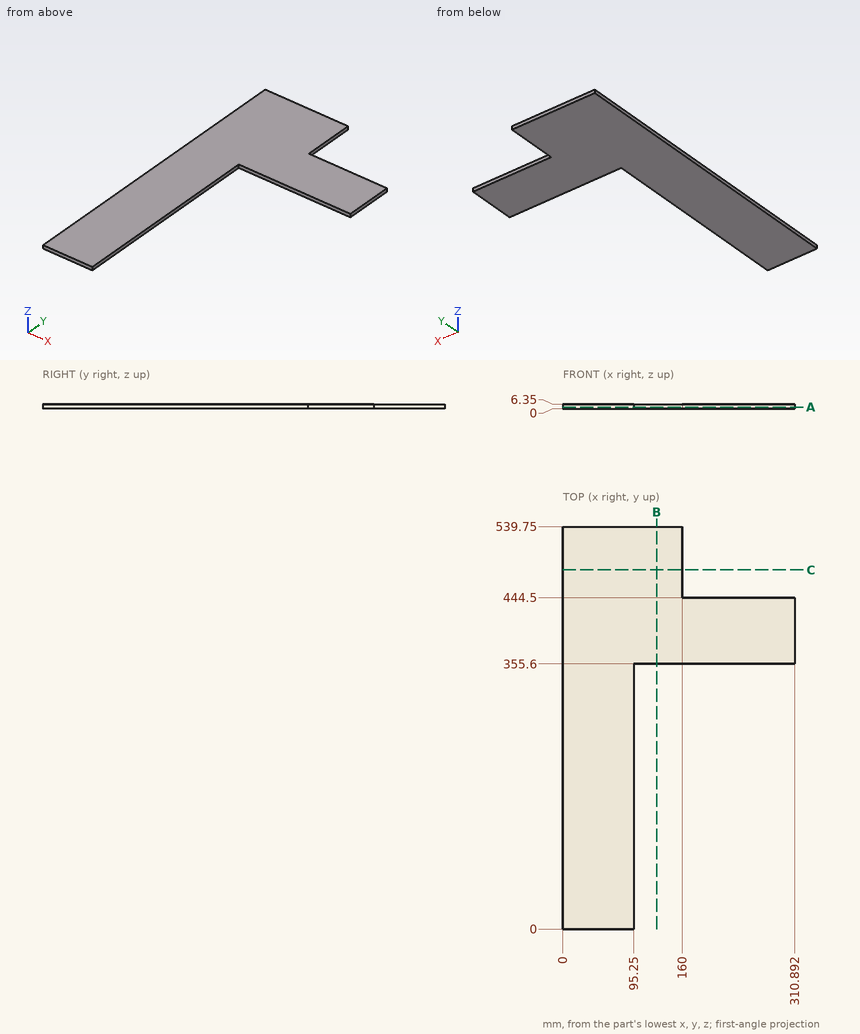
The figure shows three views and two pictorial views of one solid part (mm, origin at its lowest corner). Answer the questions. Coordinates: 2 decimals unless noted, no trailing zeros. Write each loop counter-clockwise with the first axis right and the second up, starting at its lowest first coordinate (ties: lowest second). Pieces come first, ordered by that corner, then holes. Notation, with made-up numbers: (-24, 86.5) -> (-19, 86.5) arc R10 ccw to (-19, 95.5) -> close; hole circle Ø2 at (-25, 28.5). An arc over 180 degrees is marked (long way). Answer as a JSON object with one key per item and string values.
Q1. The part is cut by section A-A on z = 2.25. Give the vertices of the cut face in (x, y).
The answers:
{"outline": "(0, 0) -> (95.25, 0) -> (95.25, 355.6) -> (310.89, 355.6) -> (310.89, 444.5) -> (160, 444.5) -> (160, 539.75) -> (0, 539.75) -> close"}
Q2. The part is cut by section B-B on x = 126. Give the vertices of the cut face in (y, z).
The answers:
{"outline": "(355.6, 0) -> (539.75, 0) -> (539.75, 6.35) -> (355.6, 6.35) -> close"}
Q3. The part is cut by section C-C on y = 482. Give the vertices of the cut face in (x, z).
The answers:
{"outline": "(0, 0) -> (160, 0) -> (160, 6.35) -> (0, 6.35) -> close"}
Q4. Flat-ended cylindrical pins translate along their axes: pin 1 Ø2 at (x, z) = (146, 3.5) entering from -Y; pin 2 Ø1.5 at (x, z) = (251.5, 2) entering from +Y; pin 3 Ø5 at (x, y) = (81.5, 381) entering from -Z. Find the tip coordinate at first contact, or state that the pin passes through.
The answers:
{"pin 1": "stops at y = 355.6", "pin 2": "stops at y = 444.5", "pin 3": "stops at z = 0"}
Q5. Consider line 1 (Y direction, x = 202, z = 5); line 2 (X direction, y = 177, z = 0.75); line 3 (Y direction, x = 148, z = 3.5). Determine where each line is inside the solid, lowest interval first. Write a range as [from, to].
The answers:
{"line 1": "y = [355.6, 444.5]", "line 2": "x = [0, 95.25]", "line 3": "y = [355.6, 539.75]"}
